Drawing for the job (mm, zero at the part's lowest x, y, z). A direction names the side the tool comes from. Give positions to 0.01 mm unless a question says otherwise; leave off trailing zeros. Loops run counter-clockwise (first coordinate to the right, second up) from the corner with the lowest first, then second, coordinate; pieces in that order, holes last. Notation, with made-up numbers: (79, 41) - (93, 41) arc R20 ccw to (93, 72) - close; hole circle Ø3 at (31.5, 10). An arc over 180 degrees is marked (long way). Return JSON: item names as keys, results as strings. Group by question number.
1) Slice it at A-A (z = 5). List the corners of the cut face in (x, y).
2) Slice it at C-C (x = 17.75). List the corners of the cut face in (y, z), and give its area (3 significant figures).
3) Drop flat-ended pins along their axis: pin 1 (4.5 mm diameter, centred on y = 6.5, z = 5, fed in from +X); pin 2 (4.5 mm diameter, centred on y = 9, z = 7, fed in from -X); pin 3 (3.5 mm diameter, centred on x = 19, z = 1.5, fed in from -Y); pin 4 (1 mm diameter, centred on y = 10, z = 2.5, fed in from -X). Give the stop position or say it passes through.
4) Slice it at B-B (y = 6.5). List the corners of the cut face in (x, z), and give its area (3 significant figures).
5) 3-axis set-ups, long thin cutter, end or side, ignore diameter. For the marked faces 4, 5 and 6: which of +Z, -Z, +X, -X, +Y, -Y reach the whole face in a straight line?
6) Slice it at D-D (z = 11). List the corners of the cut face in (x, y), and give its area (3 significant figures).
7) Drill centre lines: probe 1 along Z at (x, y) = (12.25, 6.5); probe 2 along Z at (x, y) = (16.5, 11); probe 3 along X at (y, z) = (6.75, 11.75). Where is each one in solid material? Low to high. Write a range as from..to.
8) Mould opens along Z. For the marked faces 1, 2 and 3 say: released by +Z, released by -Z, zero draft, split by the parting line, or undercut.
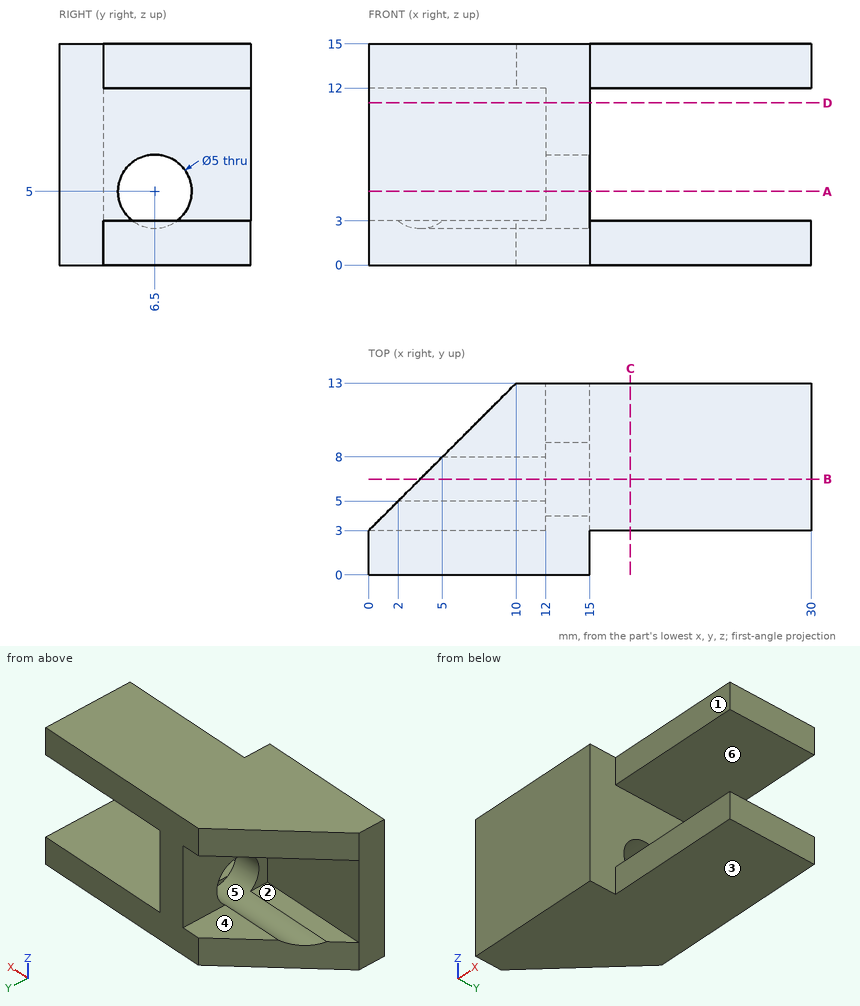
Results:
{
 "1": {"outline": "(0, 0) - (15, 0) - (15, 4) - (12, 4) - (12, 3) - (0, 3) - close; (12, 9) - (15, 9) - (15, 13) - (12, 13) - close"},
 "2": {"outline": "(3, 0) - (13, 0) - (13, 3) - (3, 3) - close; (3, 12) - (13, 12) - (13, 15) - (3, 15) - close", "area": "60.0 mm2"},
 "3": {"pin 1": "x = 30", "pin 2": "x = 12", "pin 3": "y = 3", "pin 4": "x = 6.5"},
 "4": {"outline": "(3.5, 0) - (30, 0) - (30, 3) - (15, 3) - (15, 2.5) - (3.5, 2.5) - close; (3.5, 12) - (12, 12) - (12, 7.5) - (15, 7.5) - (15, 12) - (30, 12) - (30, 15) - (3.5, 15) - close", "area": "167 mm2"},
 "5": {"face 4": "-X, +Y", "face 5": "-X", "face 6": "+X, +Y, -Y"},
 "6": {"outline": "(0, 0) - (15, 0) - (15, 13) - (12, 13) - (12, 3) - (0, 3) - close", "area": "75.0 mm2"},
 "7": {"probe 1": "0..2.5, 7.5..15", "probe 2": "0..3, 12..15", "probe 3": "12..15"},
 "8": {"face 1": "zero draft", "face 2": "undercut", "face 3": "released by -Z"}
}
